Geometry: see drawing. Coordinates: mm, zero at the bounding-box minimum. Coordinates: 2 decimals unless noted, no trailing zeros. Loops run counter-clockwise (first coordinate to the right, second up) from the corner with the lowest first, then second, coordinate; pieces in that order, holes last.
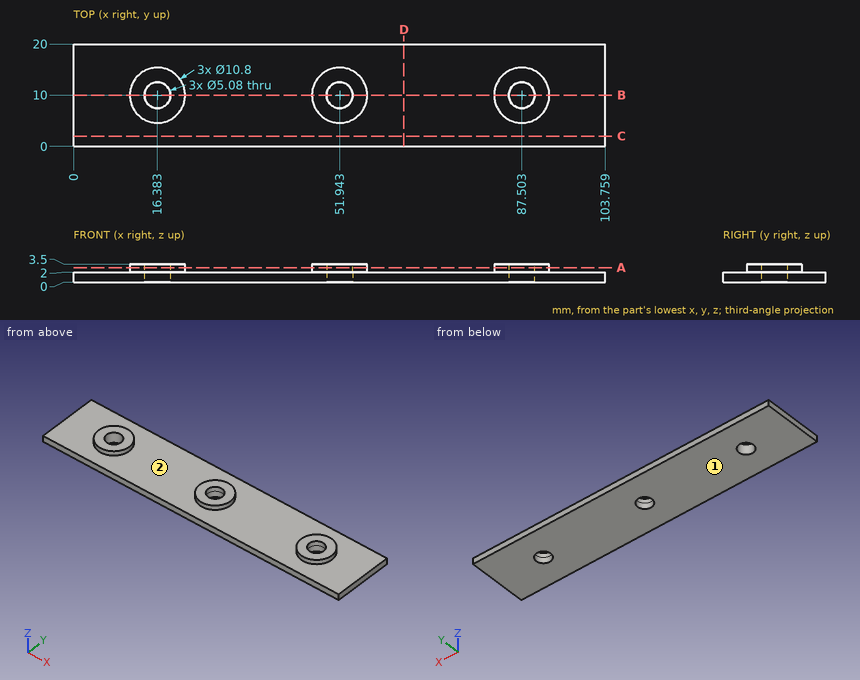
Item 1: Section query C-C (y = 2). Output: boundary loops of the cut face in (x, z).
Result:
outline: (0, 0) - (103.76, 0) - (103.76, 2) - (0, 2) - close
Item 2: Section query B-B (y = 10). Output: boundary loops of the cut face in (x, z).
Result:
outline: (0, 0) - (13.84, 0) - (13.84, 3.5) - (10.98, 3.5) - (10.98, 2) - (0, 2) - close; (18.92, 0) - (49.4, 0) - (49.4, 3.5) - (46.54, 3.5) - (46.54, 2) - (21.78, 2) - (21.78, 3.5) - (18.92, 3.5) - close; (54.48, 0) - (84.96, 0) - (84.96, 3.5) - (82.1, 3.5) - (82.1, 2) - (57.34, 2) - (57.34, 3.5) - (54.48, 3.5) - close; (90.04, 0) - (103.76, 0) - (103.76, 2) - (92.9, 2) - (92.9, 3.5) - (90.04, 3.5) - close
Item 3: Section query A-A (z = 2.9). Output: boundary loops of the cut face in (x, y), then the cut area to 3 significant figures.
Result:
outline: circle Ø10.8 at (16.38, 10); circle Ø10.8 at (51.94, 10); circle Ø10.8 at (87.5, 10); hole circle Ø5.08 at (16.38, 10); hole circle Ø5.08 at (51.94, 10); hole circle Ø5.08 at (87.5, 10)
area: 214 mm2
Item 4: Mould query, pull axis X, two halves, no side actions, for the marked faces 1 and 2. Classes: +X half, -X half, draft (parallel to the pull), parting line (faces both ways), or undercut.
Result:
face 1: draft
face 2: undercut
Item 5: Line query: L1, parallel to X at y = 10, z = 0.8; L2, parallel to Z at x = 76, y = 16.25; L3, parallel to X at y = 11.5, z = 3.35. Output: solid intervals per line, ascending.
Result:
L1: x = 0 to 13.84, 18.92 to 49.4, 54.48 to 84.96, 90.04 to 103.76
L2: z = 0 to 2
L3: x = 11.2 to 14.33, 18.43 to 21.57, 46.76 to 49.89, 53.99 to 57.13, 82.32 to 85.45, 89.55 to 92.69
Item 6: Contact query for flat-ended pins moving along their axis: P1, Ø2, axis at x = 60.5, y = 7, coming from the +Z side; P2, Ø6.5, axis at x = 87.503, y = 10, coming from the +Z side. Output: stop coordinate, or through.
Result:
P1: stops at z = 2
P2: stops at z = 3.5
Item 7: Section query D-D (x = 64.5). Output: boundary loops of the cut face in (y, z), then the cut area to 3 significant figures.
Result:
outline: (0, 0) - (20, 0) - (20, 2) - (0, 2) - close
area: 40.0 mm2
